Autodesk Inventor part; units mm, degrees
ref_plane "YZ Plane" through (0, 0, 0) normal (1, 0, 0) x (0, 1, 0)
ref_plane "XZ Plane" through (0, 0, 0) normal (0, 1, 0) x (-1, 0, 0)
ref_plane "XY Plane" through (0, 0, 0) normal (0, 0, 1) x (1, 0, 0)
sketch "スケッチ1" plane through (0, 0, 0) normal (0, 0, 1) x (1, 0, 0)
  line L0 (-26.25, 0) -> (26.25, 0) construction
  line L1 (0, -17.15) -> (0, 17.15) construction
  line L2 (-18.75, 12.25) -> (18.75, 12.25)
  line L3 (18.75, 12.25) -> (18.75, -7.25)
  line L4 (13.75, -12.25) -> (-13.75, -12.25)
  line L5 (-18.75, -7.25) -> (-18.75, 12.25)
  line L6 (-13.75, -12.25) -> (-18.75, -7.25)
  line L7 (18.75, -7.25) -> (13.75, -12.25)
  point P0 (0, 0)
  point P1 (18.75, -12.25)
  point P2 (-18.75, -12.25)
  dimension "d0" = 37.5
  dimension "d1" = 24.5
  dimension "d2" = 18.75
  dimension "d3" = 12.25
  dimension "d76" = 5
  dimension "d77" = 5
  dimension "d78" = 5
  dimension "d79" = 5
extrude "押し出し1" add sketch "スケッチ1" along normal blind 18.5
sketch "スケッチ2" plane through (0, 0, 18.5) normal (0, 0, 1) x (1, 0, 0)
  line L0 (18.75, 12.25) -> (-18.75, 12.25)
  line L1 (-18.75, 12.25) -> (-18.75, -7.25)
  line L2 (-13.75, -12.25) -> (13.75, -12.25)
  line L3 (18.75, -7.25) -> (18.75, 12.25)
  line L4 (16.75, 10.25) -> (16.75, -7.25)
  line L5 (13.75, -10.25) -> (-13.75, -10.25)
  line L6 (-16.75, -7.25) -> (-16.75, 10.25)
  line L7 (-11.5, 12.25) -> (11.5, 12.25)
  line L8 (11.5, 12.25) -> (11.5, 10.25)
  line L9 (-11.5, 10.25) -> (-11.5, 12.25)
  line L10 (-16.75, 10.25) -> (-11.5, 10.25)
  line L11 (11.5, 10.25) -> (16.75, 10.25)
  line L12 (-16.75, -7.25) -> (-13.75, -10.25)
  line L13 (16.75, -7.25) -> (13.75, -10.25)
  point P0 (-18.75, -12.25)
  point P1 (18.75, -12.25)
  point P2 (0, 0)
  dimension "d6" = 2
  dimension "d7" = 7.25
  dimension "d8" = 7.25
  dimension "d66" = 5
  dimension "d67" = 5
  dimension "d68" = 5
  dimension "d69" = 5
  dimension "d71" = 2
  dimension "d72" = 2
  dimension "d74" = 2
  dimension "d75" = 2
extrude "押し出し2" cut sketch "スケッチ2" against normal blind 16.5
sketch "スケッチ3" plane through (0, 0, 2) normal (0, 0, 1) x (1, 0, 0)
  line L0 (13.75, -10.25) -> (-13.75, -10.25)
  line L1 (-1.5, -10.25) -> (1.5, -10.25)
  line L2 (1.5, -10.25) -> (1.5, -1.75)
  line L3 (1.5, -1.75) -> (-1.5, -1.75)
  line L4 (-1.5, -1.75) -> (-1.5, -10.25)
  point P0 (0, 0)
  dimension "d11" = 3
  dimension "d12" = 8.5
  dimension "d13" = 1.5
extrude "押し出し3" add sketch "スケッチ3" along normal blind 3.5
sketch "スケッチ4" plane through (-16.75, 10.25, 18.5) normal (0, -1, 0) x (1, 0, 0)
  line L0 (0, 0) -> (5.25, 0)
  line L1 (5.25, 0) -> (5.25, -16.5)
  point P0 (16.75, -18.5)
  point P1 (2.75, -6.25)
  dimension "d16" = 6.25
  dimension "d50" = 2.5
hole "穴1" at (-14, 10.25, 12.25) direction (0, 1, 0) diameter 1.6 end through all
mirror "ミラー1" about plane through (0, 0, 0) normal (1, 0, 0) of "穴1"
sketch "スケッチ5" plane through (-18.75, -12.25, 0) normal (0, -1, 0) x (1, 0, 0)
  circle A0 centre (4.75, 12.25) radius 0.8
  line L0 (5, 18.5) -> (32.5, 18.5)
  point P0 (18.75, 0)
  point P1 (12.75, 12.25)
  point P2 (37.5, 18.5)
  point P3 (0, 18.5)
  dimension "d25" = 8
  dimension "d60" = 6.25
hole "穴2" at (-6, -12.25, 12.25) direction (0, 1, 0) diameter 1.6 end through all
sketch "スケッチ6" plane through (0, 0, 2) normal (0, 0, 1) x (1, 0, 0)
  line L0 (-1.5, -10.25) -> (-13.75, -10.25)
  point P0 (0, 0)
  point P1 (0, 5.75)
  dimension "d33" = 16
hole "穴3" at (0, 5.75, 2) direction (0, 0, -1) diameter 2.5 end through all
sketch "スケッチ7" plane through (0, 0, 2) normal (0, 0, 1) x (1, 0, 0)
  circle A0 centre (0, 5.75) radius 1.25
  point P0 (0, 0)
  point P1 (-6.5, 5.75)
  point P2 (-12.5, 5.75)
  dimension "d41" = 6.5
  dimension "d42" = 12.5
hole "穴4" at (-6.5, 5.75, 2) at (-12.5, 5.75, 2) direction (0, 0, -1) diameter 1.6 end through all
mirror "ミラー2" about plane through (0, 0, 0) normal (1, 0, 0) of "穴4"
sketch "スケッチ8" plane through (0, 0, 2) normal (0, 0, 1) x (1, 0, 0)
  line L0 (-16.75, 10.25) -> (-11.5, 10.25)
  line L1 (-16.75, -10.25) -> (-16.75, 10.25)
  line L2 (-16.75, 7.25) -> (-11.5, 7.25)
  line L3 (-11.5, 7.25) -> (-11.5, 5.25)
  line L4 (-11.5, 5.25) -> (-16.75, 5.25)
  line L5 (-16.75, 5.25) -> (-16.75, 7.25)
  point P0 (-13.75, -10.25)
  point P1 (0, 0)
  dimension "d51" = 2
  dimension "d52" = 5.25
  dimension "d53" = 3
extrude "押し出し4" add sketch "スケッチ8" along normal blind 16.5
sketch "スケッチ9" plane through (-16.75, 5.25, 2) normal (0, -1, 0) x (1, 0, 0)
  circle A0 centre (2.75, 10.25) radius 0.8
  point P0 (16.75, -2)
extrude "押し出し5" cut sketch "スケッチ9" against normal blind 3
mirror "ミラー3" about plane through (0, 0, 0) normal (1, 0, 0) of "押し出し4"
mirror "ミラー4" about plane through (0, 0, 0) normal (1, 0, 0) of "押し出し5"
sketch "スケッチ10" plane through (-18.75, 12.25, 0) normal (0, 1, 0) x (1, 0, 0)
  circle A0 centre (4.75, -12.25) radius 0.8
  line L0 (7.25, -18.5) -> (7.25, -2)
  line L1 (4.75, -11.45) -> (7.25, -11.45)
  line L2 (7.25, -11.45) -> (7.25, -13.05)
  line L3 (7.25, -13.05) -> (4.75, -13.05)
  line L4 (4.75, -13.05) -> (4.75, -11.45)
  point P0 (18.75, 0)
extrude "押し出し6" cut sketch "スケッチ10" against normal blind 10 contours A0 L4 | A0 L1 L0 L3 picked at (4.8657, -12.0097)
mirror "ミラー5" about plane through (0, 0, 0) normal (1, 0, 0) of "押し出し6"
equation "\"d2\" = 0.5 * d0"
equation "\"d3\" = 0.5 * d1"
equation "\"d8\" = d7"
properties part number "case-new"
Check sheet for the modelled part. Datum: model origin and axes. Units: mm. A direction names the side the tool comes from. Give positions to 0.01 mm unless a question says otherwise; leave off trailing zeros. Loops run counter-clockwise (first coordinate to the right, second up) from the corner with the lowest first, then second, coordinate; pieces in that order, holes last. Notation, with made-up numbers: M 74,19 L 101,19 A25 cw 101,35 Z; hole C 5.25,-26.75 d8. An arc over 180 degrees is marked long. Answer as a JSON object with one key per item and string values. Group by question number.
Q1. Cross-section at D-D on y = 2. Record the cut outline in (x, z), then the cut area to 3 significant figures.
Q2. Go/stop test with flat-tipped pins: P1, Ø4, axis at x = 15, z = 14, coming from the -Y side; P2, Ø5, axis at x = -1.5, z = 12.5, coming from the +Y side; P3, Ø5, axis at x = -1.5, z = 5, coming from the +Y side. Record where each tip stops, or that it passes through.
Q3. Cross-section at C-C on x = -16. Record the cut outline in (y, z), then the cut area to 4 significant figures.
Q4. Material ranges on line 1 along X through (y, z) = (5.75, 0.65); line 2 along Y through (x, z) = (13, 10); line 3 along X through (y, z) = (7.5, 2.25), recorded low to high. Write a range as [from, to].
Q5. Cross-section at A-A on x = 12.5. Record the cut outline in (y, z).
Q6. Access from +Z, -Z, +X, -X, +Y, -Y to the whole of each face (thin tool, end or side, straight path). Record for faces 1 (the flat face through (-13, 6, 2)), 2 (the flat face through (11.5, 11, 7)), 3 (the flat face through (-13, 6, 13.05)).
Q7. Cross-section at B-B on z = 7. Record the cut outline in (x, y).
Q8. Release check for a two-part mould opening along Z. For faces 4 (the cylindrical face through (14.8, 6.2, 12.2)), 5 (the flat face through (0, -6, 5.5)), 6 (the flat face through (-16.75, 9, 10)) record: released by +Z, released by -Z, zero draft, split by the parting line, or undercut.
Evaluation:
{
 "1": {"outline": "M -18.75,0 L 18.75,0 L 18.75,18.5 L 16.75,18.5 L 16.75,2 L -16.75,2 L -16.75,18.5 L -18.75,18.5 Z", "area": "141 mm2"},
 "2": {"P1": "stops at y = -12.25", "P2": "stops at y = -10.25", "P3": "stops at y = -1.75"},
 "3": {"outline": "M -10,0 L 12.25,0 L 12.25,18.5 L 10.25,18.5 L 10.25,2 L 7.25,2 L 7.25,18.5 L 5.25,18.5 L 5.25,2 L -8,2 L -8,18.5 L -10,18.5 Z", "area": "143.5 mm2"},
 "4": {"line 1": "x = [-18.75, -13.3], [-11.7, -7.3], [-5.7, -1.25], [1.25, 5.7], [7.3, 11.7], [13.3, 18.75]", "line 2": "y = [-12.25, -10.25], [5.25, 7.25], [10.25, 12.25]", "line 3": "x = [-18.75, -16.75], [16.75, 18.75]"},
 "5": {"outline": "M -12.25,0 L 4.95,0 L 4.95,2 L -10.25,2 L -10.25,18.5 L -12.25,18.5 Z; M 5.25,2 L 6.55,2 L 6.55,0 L 12.25,0 L 12.25,11.45 L 10.25,11.45 L 10.25,2 L 7.25,2 L 7.25,11.45 L 5.25,11.45 Z; M 5.25,13.05 L 7.25,13.05 L 7.25,18.5 L 5.25,18.5 Z; M 10.25,13.05 L 12.25,13.05 L 12.25,18.5 L 10.25,18.5 Z"},
 "6": {"face 1": "-Z", "face 2": "+Z, +Y", "face 3": "+Y"},
 "7": {"outline": "M -18.75,-7.25 L -13.75,-12.25 L 13.75,-12.25 L 18.75,-7.25 L 18.75,12.25 L 11.5,12.25 L 11.5,10.25 L 16.75,10.25 L 16.75,7.25 L 11.5,7.25 L 11.5,5.25 L 16.75,5.25 L 16.75,-7.25 L 13.75,-10.25 L -13.75,-10.25 L -16.75,-7.25 L -16.75,5.25 L -11.5,5.25 L -11.5,7.25 L -16.75,7.25 L -16.75,10.25 L -11.5,10.25 L -11.5,12.25 L -18.75,12.25 Z"},
 "8": {"face 4": "undercut", "face 5": "released by +Z", "face 6": "zero draft"}
}
